```python
from build123d import *

# Parameters (mm, degrees)
BOSS_EXTRUDE3_DEPTH = 1.5
SKETCH3_R           = 1.5
CUT_EXTRUDE6_DEPTH  = 1.5


with BuildPart() as part:
    # Sketch5 → Boss-Extrude3 (new body)
    with BuildSketch(Plane(origin=(0, 0, 0), x_dir=(1, 0, 0), z_dir=(0, 1, 0))):
        Polygon((-31.936172748, 32.164122013), (-37.46862037, 25.951620882), (-37.46862037, 14.483050574), (-39.885792802, 11.768757102), (-39.885792802, -22.264531804), (-37.547976629, -24.602347977), (-37.547976629, -31.835877987), (-31.61237508, -31.835877987), (36.114207198, -31.835877987), (36.114207198, 32.164122013), align=None)
    extrude(amount=BOSS_EXTRUDE3_DEPTH)

    # Sketch3 → Cut-Extrude6 (cut)
    with BuildSketch(Plane(origin=(0, 0, 0), x_dir=(1, 0, 0), z_dir=(0, 1, 0))):
        with Locations((-34.085940204, 9.171489798)):
            Circle(SKETCH3_R)
        with Locations((-34.085040269, -18.784732287)):
            Circle(SKETCH3_R)
        with Locations((17.126200612, 24.50342873)):
            Circle(SKETCH3_R)
        with Locations((18.50498177, -23.809750535)):
            Circle(SKETCH3_R)
    extrude(amount=CUT_EXTRUDE6_DEPTH, mode=Mode.SUBTRACT)


solid = part.part
```
The model under review builds one solid part; all positions refer to its coordinate system, in mm. A direction names the side the tool comes from. Coordinates: 2 decimals unless noted, no trailing zeros. Write each loop counter-clockwise with the first axis right and the second up, starting at its lowest first coordinate (ties: lowest second). Pieces come first, ordered by that corner, then holes. Notation, with made-up numbers: (47.25, 47) - (81.25, 47) arc R6 ccw to (81.25, 52) - close; hole circle Ø6 at (76.25, 78.5). An arc over 180 degrees is marked (long way). Answer in a Markdown table with one row per item. Add a question column.
Q1. For faces 5 (the face through (19.891, 0.74, 24.384)), 6 (the face through (-37.548, 1, 28)), 7 (the face through (-37.469, 1, -20)), list the 3-axis set-ups (+Z, -Z, +X, -X, +Y, -Y) from which the entire face can be reached by the end or side of a thin tool; tool diameter is ignored.
Q2. Clearance check with flat-ended pins moving along their axes: pin 1 (5 mm diameter, centred on x = 11.5, z = -14, fed in from -Y); pin 2 (0.8 mm diameter, centred on y = 0.5, z = -22.5, fed in from -X). State where each tip first meets the part, or that it passes through.
Q3. Draft analysis for pull direction Z (two halves, no side actions). For faces 1 (the face through (17, 1, -26)), 2 (the face through (-2, 1.5, -1)), 3 (the face through (-1, 1, 31.836)), 4 (the face through (-34.664, 0.74, -29.101)), state which applies: +Z half, -Z half, draft (parallel to the pull), parting line (faces both ways), or undercut.
Q4. Consider section A-A on y = 0.8. Give the boundary of the cut face in (x, z).
Q5. To check wall thickness, follow line 1 along Z through (x, y) = (-33, 0.1); line 2 along Z through (x, y) = (19.5, 1.1); line 3 along X through (y, z) = (0.6, 18). State the ranges of each line that lie inside material, in increasing order. Write a range as from..to.
Answers below:
| question | item | result |
|---|---|---|
| 1 | face 5 | +Y, -Y |
| 1 | face 6 | +Z, -X, +Y, -Y |
| 1 | face 7 | -Z, -X, +Y, -Y |
| 2 | pin 1 | y = 0 |
| 2 | pin 2 | x = -37.47 |
| 3 | face 1 | undercut |
| 3 | face 2 | draft |
| 3 | face 3 | +Z half |
| 3 | face 4 | -Z half |
| 4 | outline | (-39.89, -11.77) - (-37.47, -14.48) - (-37.47, -25.95) - (-31.94, -32.16) - (36.11, -32.16) - (36.11, 31.84) - (-37.55, 31.84) - (-37.55, 24.6) - (-39.89, 22.26) - close; hole circle Ø3 at (-34.09, -9.17); hole circle Ø3 at (-34.09, 18.78); hole circle Ø3 at (17.13, -24.5); hole circle Ø3 at (18.5, 23.81) |
| 5 | line 1 | -30.97..-10.21, -8.14..17.75, 19.82..31.84 |
| 5 | line 2 | -32.16..22.69, 24.93..31.84 |
| 5 | line 3 | -39.89..-35.36, -32.81..36.11 |
